Input: part model. Units: mm. Frame: model coordinates. Round coordinates to 2 decimals unless told otherwise and drop trailing zeros. Loops run counter-clockwise (first coordinate to the right, second up) from the corner with the lowest first, then second, coordinate; pieces in that order, holes last. Notation, with made-up numbers: (12, -5) - (30, -5) arc R28 cw to (30, 18) - close; hole circle Ø2 at (-37, -31). An arc over 180 degrees is marked (long way). Write each question's results on one line, items separated by ' | '.
from build123d import *

# Parameters (mm, degrees)
SKETCH_1_W          = 10
SKETCH_1_H          = 12
EXTRUDE_1_DEPTH     = 0.6
SKETCH_2_W          = 10
SKETCH_2_H          = 12
CUT_EXTRUDE_1_DEPTH = 0.1
SKETCH_4_W          = 10
SKETCH_4_H          = 12
CUT_EXTRUDE_3_DEPTH = 0.05
FILLET_1_R          = 0.2


with BuildPart() as part:
    # 草图1 → 凸台-拉伸1 (new body)
    with BuildSketch(Plane.XY):
        with Locations((-0.081339713, 0.803827751)):
            Rectangle(SKETCH_1_W, SKETCH_1_H)
    extrude(amount=EXTRUDE_1_DEPTH)

    # 草图2 → 切除-拉伸1 (cut)
    with BuildSketch(Plane(origin=(0, 0, 0), x_dir=(-1, 0, 0), z_dir=(0, 0, -1))):
        with Locations((0.081339713, 0.803827751)):
            Rectangle(SKETCH_2_W, SKETCH_2_H)
        with BuildLine():
            Line((-2.712551899, 5.7889264), (2.884041266, 5.7889264))
            ThreePointArc((2.884041266, 5.7889264), (3.591148047, 5.496033181), (3.884041266, 4.7889264))
            Line((3.884041266, 4.7889264), (3.884041266, -3.115928634))
            ThreePointArc((3.884041266, -3.115928634), (3.591148047, -3.823035415), (2.884041266, -4.115928634))
            Line((2.884041266, -4.115928634), (-2.712551899, -4.115928634))
            ThreePointArc((-2.712551899, -4.115928634), (-3.419658681, -3.823035415), (-3.712551899, -3.115928634))
            Line((-3.712551899, -3.115928634), (-3.712551899, 4.7889264))
            ThreePointArc((-3.712551899, 4.7889264), (-3.419658681, 5.496033181), (-2.712551899, 5.7889264))
        make_face(mode=Mode.SUBTRACT)
    extrude(amount=-CUT_EXTRUDE_1_DEPTH, mode=Mode.SUBTRACT)

    # 草图4 → 切除-拉伸3 (cut, symmetric)
    with BuildSketch(Plane.XY.offset(0.3)):
        with Locations((-0.081339713, 0.803827751)):
            Rectangle(SKETCH_4_W, SKETCH_4_H)
        Polygon((0, 1.877578929), (-0.909343659, 0.803827751), (0, -0.374397758), (0.997821393, 0.803827751), align=None, mode=Mode.SUBTRACT)
    extrude(amount=CUT_EXTRUDE_3_DEPTH, both=True, mode=Mode.SUBTRACT)

    # 圆角1
    fillet_1_edges = [part.edges().sort_by_distance(p)[0] for p in [
        (-5.081339713, 6.803827751, 0.175),
        (4.918660287, 6.803827751, 0.175),
        (4.918660287, -5.196172249, 0.175),
        (-5.081339713, -5.196172249, 0.175),
        (-5.081339713, 6.803827751, 0.475),
        (4.918660287, 6.803827751, 0.475),
        (4.918660287, -5.196172249, 0.475),
        (-5.081339713, -5.196172249, 0.475),
    ]]
    fillet(fillet_1_edges, radius=FILLET_1_R)


solid = part.part
1. Section query C-C, the plane x = -2.75. Output: boundary loops of the cut face in (y, z), plus the area to 3 significant figures.
Answer:
outline: (-5.2, 0.1) - (-4.12, 0.1) - (-4.12, 0) - (5.79, 0) - (5.79, 0.1) - (6.8, 0.1) - (6.8, 0.25) - (-5.2, 0.25) - close; (-5.2, 0.35) - (6.8, 0.35) - (6.8, 0.6) - (-5.2, 0.6) - close | area: 5.79 mm^2
2. Line query: line 1 (Y direction, x = 4.75, z = 0.15). Output: solid intervals per line, ascending. Write a range as [from, to].
Answer:
line 1: [-5.19, 6.8]
3. Section query A-A, the plane y = -1.75. Output: boundary loops of the cut face in (x, z).
Answer:
outline: (-5.08, 0.1) - (-3.88, 0.1) - (-3.88, 0) - (3.71, 0) - (3.71, 0.1) - (4.92, 0.1) - (4.92, 0.25) - (-5.08, 0.25) - close; (-5.08, 0.35) - (4.92, 0.35) - (4.92, 0.6) - (-5.08, 0.6) - close
4. Section query B-B, the plane x = 4. Output: boundary loops of the cut face in (y, z).
Answer:
outline: (-5.2, 0.1) - (6.8, 0.1) - (6.8, 0.25) - (-5.2, 0.25) - close; (-5.2, 0.35) - (6.8, 0.35) - (6.8, 0.6) - (-5.2, 0.6) - close
5. Section query D-D, the plane x = 0.75. Output: boundary loops of the cut face in (y, z), plus the area to 3 significant figures.
Answer:
outline: (-5.2, 0.1) - (-4.12, 0.1) - (-4.12, 0) - (5.79, 0) - (5.79, 0.1) - (6.8, 0.1) - (6.8, 0.25) - (1.07, 0.25) - (1.07, 0.35) - (6.8, 0.35) - (6.8, 0.6) - (-5.2, 0.6) - (-5.2, 0.35) - (0.51, 0.35) - (0.51, 0.25) - (-5.2, 0.25) - close | area: 5.85 mm^2
